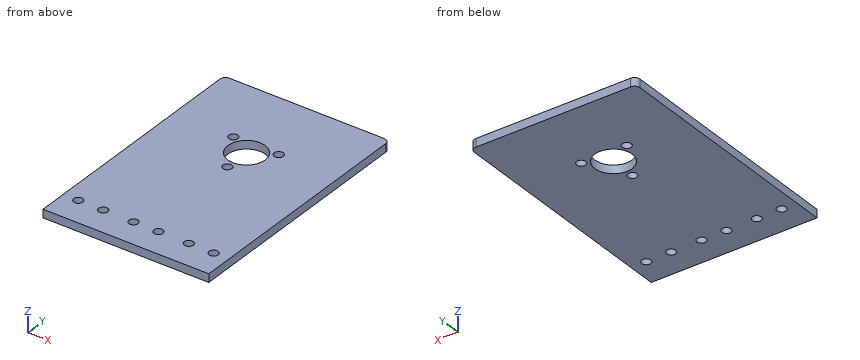
from build123d import *

# Parameters (mm, degrees)
SKETCH_1_W          = 60
SKETCH_1_H          = 90
EXTRUDE_1_DEPTH     = 3
SKETCH_2_R          = 1.65
CUT_EXTRUDE_1_DEPTH = 3
SKETCH_3_R          = 1.65
CUT_EXTRUDE_2_DEPTH = 3
SKETCH_4_R          = 6.75
CUT_EXTRUDE_3_DEPTH = 3
FILLET_1_R          = 2


with BuildPart() as part:
    # 草图1 → 凸台-拉伸1 (new body)
    with BuildSketch(Plane.XY):
        Rectangle(SKETCH_1_W, SKETCH_1_H)
    extrude(amount=EXTRUDE_1_DEPTH)

    # 草图2 → 切除-拉伸1 (cut)
    with BuildSketch(Plane.XY.offset(3)):
        with Locations((0, 5.5)):
            Circle(SKETCH_2_R)
        with Locations((-8.227241336, 19.75)):
            Circle(SKETCH_2_R)
        with Locations((8.227241336, 19.75)):
            Circle(SKETCH_2_R)
    extrude(amount=-CUT_EXTRUDE_1_DEPTH, mode=Mode.SUBTRACT)

    # 草图3 → 切除-拉伸2 (cut)
    with BuildSketch(Plane.XY.offset(3)):
        with Locations((4.5, -35)):
            Circle(SKETCH_3_R)
        with Locations((-4.5, -35)):
            Circle(SKETCH_3_R)
        with Locations((24.5, -35)):
            Circle(SKETCH_3_R)
        with Locations((15.5, -35)):
            Circle(SKETCH_3_R)
        with Locations((-24.5, -35)):
            Circle(SKETCH_3_R)
        with Locations((-15.5, -35)):
            Circle(SKETCH_3_R)
    extrude(amount=-CUT_EXTRUDE_2_DEPTH, mode=Mode.SUBTRACT)

    # 草图4 → 切除-拉伸3 (cut)
    with BuildSketch(Plane.XY.offset(3)):
        with Locations((0, 15)):
            Circle(SKETCH_4_R)
    extrude(amount=-CUT_EXTRUDE_3_DEPTH, mode=Mode.SUBTRACT)

    # 圆角1
    fillet_1_edges = [part.edges().sort_by_distance(p)[0] for p in [
        (-30, 45, 1.5),
        (30, 45, 1.5),
    ]]
    fillet(fillet_1_edges, radius=FILLET_1_R)


solid = part.part
Verification items for the finished model (mm, model axes). Coordinates: 2 decimals unless noted, no trailing zeros. Order: outer loops, then holes, each group sorted by start corner. A loop starts at its lowest first (then second) coordinate and runs counter-clockwise, first axis right, second up. Notation, with made-up numbers: M 60,8.5 L 89,8.5 A12 cw 89,17.5 Z; hole C 47.25,21 d11. An arc over 180 degrees is marked long. One line per item, written item: value. Start each with the question number.
Item 1: Depth check by flat-ended pin: P1, Ø2.5, axis at x = 24.5, y = -35, coming from the +Z side. Enter the tip coordinate at first touch or a pass-through.
Item 2: Thickness scan on probe 1 along Y at (x, z) = (24.5, 2.1); probe 2 along X at (y, z) = (20.5, 0.7); probe 3 along Y at (x, z) = (4.5, 1.3). Record the ranges inside material, lowest first.
Item 3: Sectioned sample at C-C on z = 0.7. Give the number of separate pieces and of enclosed holes in the cut face, then the cut area to 3 significant figures.
Item 4: Sectioned sample at D-D on x = 0. Record the cut outline in (y, z).
Item 5: Sectioned sample at B-B on y = 5.5. Record the cut outline in (x, z).
Item 6: Sectioned sample at A-A on y = -35. Record the cut outline in (x, z), then the cut area to 3 significant figures.
Calculated:
1. P1: through
2. probe 1: -45 to -36.65, -33.35 to 45
2. probe 2: -30 to -9.7, -6.76 to -3.91, 3.91 to 6.76, 9.7 to 30
2. probe 3: -45 to -36.65, -33.35 to 9.97, 20.03 to 45
3. separate pieces: 1
3. enclosed holes: 10
3. area: 5,180 mm^2
4. outline: M -45,0 L 3.85,0 L 3.85,3 L -45,3 Z; M 7.15,0 L 8.25,0 L 8.25,3 L 7.15,3 Z; M 21.75,0 L 45,0 L 45,3 L 21.75,3 Z
5. outline: M -30,0 L -1.65,0 L -1.65,3 L -30,3 Z; M 1.65,0 L 30,0 L 30,3 L 1.65,3 Z
6. outline: M -30,0 L -26.15,0 L -26.15,3 L -30,3 Z; M -22.85,0 L -17.15,0 L -17.15,3 L -22.85,3 Z; M -13.85,0 L -6.15,0 L -6.15,3 L -13.85,3 Z; M -2.85,0 L 2.85,0 L 2.85,3 L -2.85,3 Z; M 6.15,0 L 13.85,0 L 13.85,3 L 6.15,3 Z; M 17.15,0 L 22.85,0 L 22.85,3 L 17.15,3 Z; M 26.15,0 L 30,0 L 30,3 L 26.15,3 Z
6. area: 121 mm^2
